The listing builds one solid part. Answer for the finished solid, in the listing's coordinates (mm). Give positions to 0.01 mm unless a question says otherwise; leave off trailing zeros. Loops run counter-clockwise (first coordinate to the right, second up) from the corner with the lowest first, then second, coordinate; pieces in that order, holes last. Notation, with made-up numbers: M 32,45 L 87,45 A30 cw 87,67 Z; hole C 65,9 d10. An arc over 180 degrees is marked long. Return JSON: item names as keys, results as strings.
from build123d import *

# Parameters (mm, degrees)
SKETCH001_R       = 108
SKETCH001_R_2     = 86.75
SKETCH001_R_3     = 2.5
PAD_DEPTH         = 10
SKETCH_R          = 1.5
POCKET_DEPTH      = 10.001
POCKET_DEPTH_BACK = 0.001


with BuildPart() as part:
    # Sketch001 → Pad (new body)
    with BuildSketch(Plane(origin=(0, 0, 0), x_dir=(1, 0, 0), z_dir=(0, 0, -1))):
        Circle(SKETCH001_R)
        Circle(SKETCH001_R_2, mode=Mode.SUBTRACT)
        with Locations((38.651027, 93.311833)):
            Circle(SKETCH001_R_3, mode=Mode.SUBTRACT)
        with Locations((93.311833, 38.651027)):
            Circle(SKETCH001_R_3, mode=Mode.SUBTRACT)
        with Locations((93.311833, -38.651027)):
            Circle(SKETCH001_R_3, mode=Mode.SUBTRACT)
        with Locations((38.651027, -93.311833)):
            Circle(SKETCH001_R_3, mode=Mode.SUBTRACT)
        with Locations((-38.651027, 93.311833)):
            Circle(SKETCH001_R_3, mode=Mode.SUBTRACT)
        with Locations((-93.311833, 38.651027)):
            Circle(SKETCH001_R_3, mode=Mode.SUBTRACT)
        with Locations((-93.311833, -38.651027)):
            Circle(SKETCH001_R_3, mode=Mode.SUBTRACT)
        with Locations((-38.651027, -93.311833)):
            Circle(SKETCH001_R_3, mode=Mode.SUBTRACT)
    extrude(amount=PAD_DEPTH)

    # Sketch → Pocket (cut, two sides)
    with BuildSketch(Plane.XY) as pocket_sk:
        with Locations((64.346717, 64.346717)):
            Circle(SKETCH_R)
        with Locations((0, 91)):
            Circle(SKETCH_R)
        with Locations((91, 0)):
            Circle(SKETCH_R)
        with Locations((64.346717, -64.346717)):
            Circle(SKETCH_R)
        with Locations((0, -91)):
            Circle(SKETCH_R)
        with Locations((-91, 0)):
            Circle(SKETCH_R)
        with Locations((-64.346717, -64.346717)):
            Circle(SKETCH_R)
        with Locations((-64.346717, 64.346717)):
            Circle(SKETCH_R)
    extrude(amount=-POCKET_DEPTH, mode=Mode.SUBTRACT)
    extrude(pocket_sk.sketch, amount=POCKET_DEPTH_BACK, mode=Mode.SUBTRACT)


solid = part.part
(1) The part is cut by section C-C (x = 8.5). Determine the outline of the cut face in (y, z).
Values follow:
{"outline": "M -107.66,-10 L -86.33,-10 L -86.33,0 L -107.66,0 Z; M 86.33,-10 L 107.66,-10 L 107.66,0 L 86.33,0 Z"}
(2) Determine the mould class of faces 1 (the cylindrical face through (-23.412, 105.432, -4.93)), 2 (the cylindrical face through (91.33, -37.13, -4.93)), 3 (the flat face through (-81, -33, -10)) for opening direction X: released by +X, released by -X, zero draft, split by the parting line, or undercut.
Values follow:
{"face 1": "split by the parting line", "face 2": "undercut", "face 3": "zero draft"}
(3) The part is cut by section B-B (z = -4). Give the number of separate pieces and of enclosed holes in the cut face, and give its area (3 significant figures).
Values follow:
{"separate pieces": "1", "enclosed holes": "17", "area": "12,800 mm²"}
(4) Given pin 1 (4 mm diameter, centred on x = -38.65, y = 93.31, fed in from -Z); pin 2 (4 mm diameter, centred on x = -74.5, z = -2, fed in from -Y); pin 3 (5 mm diameter, centred on y = 28, z = -5, fed in from +X); pin 4 (6 mm diameter, centred on y = 53.5, z = -8.5, fed in from -X), each flat-ended and moving along its own axis, determine where each tip first touches the part or whether it passes through.
Values follow:
{"pin 1": "through", "pin 2": "y = -80.05", "pin 3": "x = 104.95", "pin 4": "x = -95.47"}
(5) The part is cut by section A-A (x = 45). Determine the outline of the cut face in (y, z).
Values follow:
{"outline": "M -98.18,-10 L -74.17,-10 L -74.17,0 L -98.18,0 Z; M 74.17,-10 L 98.18,-10 L 98.18,0 L 74.17,0 Z"}
(6) Straight lines are drawn through the part: line 1 along Y through (x, z) = (0, -2.5); line 2 along Y through (x, z) = (64, -1.25); line 3 along Y through (x, z) = (33, -4.25). For each, find the intervals that lie inside material, in ascending order.
Values follow:
{"line 1": "-108 to -92.5, -89.5 to -86.75, 86.75 to 89.5, 92.5 to 108", "line 2": "-86.99 to -65.81, -62.89 to -58.56, 58.56 to 62.89, 65.81 to 86.99", "line 3": "-102.83 to -80.23, 80.23 to 102.83"}
